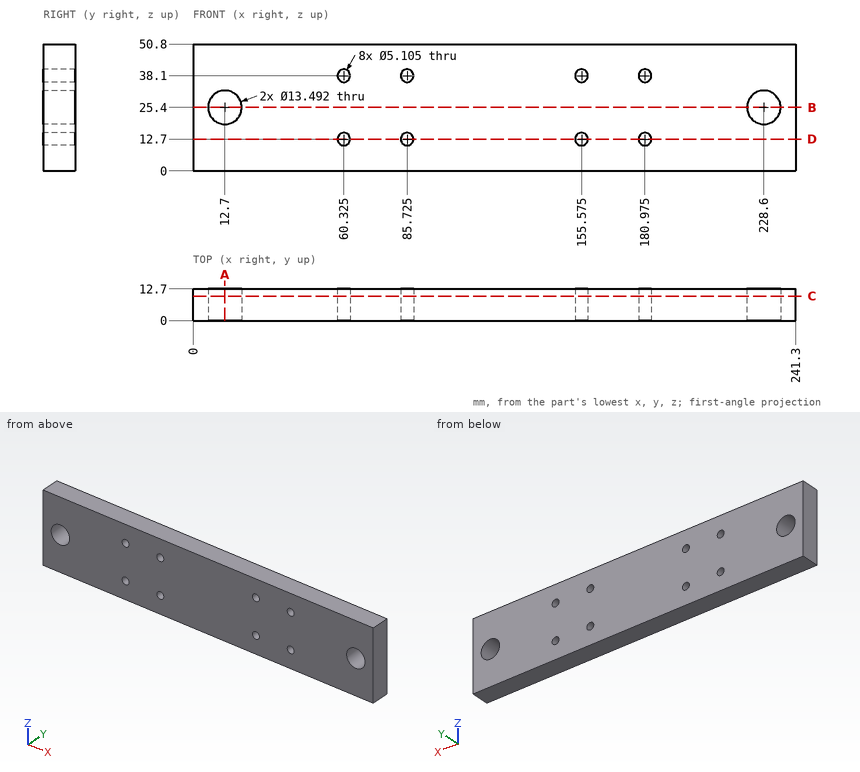
Check sheet for the drawn part. Datum: minimum x, y, z corner. Units: mm. Give positions to 0.01 mm unless a question says otherwise; leave off trailing zeros. Order: outer loops, then holes, each group sorted by start corner. A loop starts at its lowest first (then second) coordinate and runs counter-clockwise, first axis right, second up.
1. Sectioned sample at C-C (y = 9.75). State how many separate pieces and enclosed holes the cut face has, then the cut area to 3 significant figures.
Completed:
separate pieces: 1
enclosed holes: 10
area: 11,800 mm2
2. Sectioned sample at A-A (x = 12.7). Record the boundary of the cut face in (y, z).
Completed:
outline: (0, 0) - (12.7, 0) - (12.7, 18.65) - (0, 18.65) - close; (0, 32.15) - (12.7, 32.15) - (12.7, 50.8) - (0, 50.8) - close
3. Sectioned sample at B-B (z = 25.4). Record the boundary of the cut face in (x, y), then the cut area to 3 significant figures.
Completed:
outline: (0, 0) - (5.95, 0) - (5.95, 12.7) - (0, 12.7) - close; (19.45, 0) - (221.85, 0) - (221.85, 12.7) - (19.45, 12.7) - close; (235.35, 0) - (241.3, 0) - (241.3, 12.7) - (235.35, 12.7) - close
area: 2,720 mm2
4. Sectioned sample at D-D (z = 12.7). Record the boundary of the cut face in (x, y).
Completed:
outline: (0, 0) - (57.77, 0) - (57.77, 12.7) - (0, 12.7) - close; (62.88, 0) - (83.17, 0) - (83.17, 12.7) - (62.88, 12.7) - close; (88.28, 0) - (153.02, 0) - (153.02, 12.7) - (88.28, 12.7) - close; (158.13, 0) - (178.42, 0) - (178.42, 12.7) - (158.13, 12.7) - close; (183.53, 0) - (241.3, 0) - (241.3, 12.7) - (183.53, 12.7) - close
5. Scan lines: line 1 (X direction, y = 9.5, z = 38.1); line 2 (Z direction, x = 12.7, y = 5.25); line 3 (X direction, y = 4.5, z = 25.4). Record each from-to range of solid material in increasing order.
Completed:
line 1: x = 0 to 57.77, 62.88 to 83.17, 88.28 to 153.02, 158.13 to 178.42, 183.53 to 241.3
line 2: z = 0 to 18.65, 32.15 to 50.8
line 3: x = 0 to 5.95, 19.45 to 221.85, 235.35 to 241.3
